For this review, use the dimensioned drawing (mm, ordinates from the lowest corner) and the shaded views. A direction names the side the tool comes from. Give positions to 0.01 mm unless a question says otherwise; leave off trailing zeros. Order: outer loops, then holes, each group sorted by start corner. A loop starts at its lowest first (then second) coordinate and runs counter-clockwise, first axis right, second up.
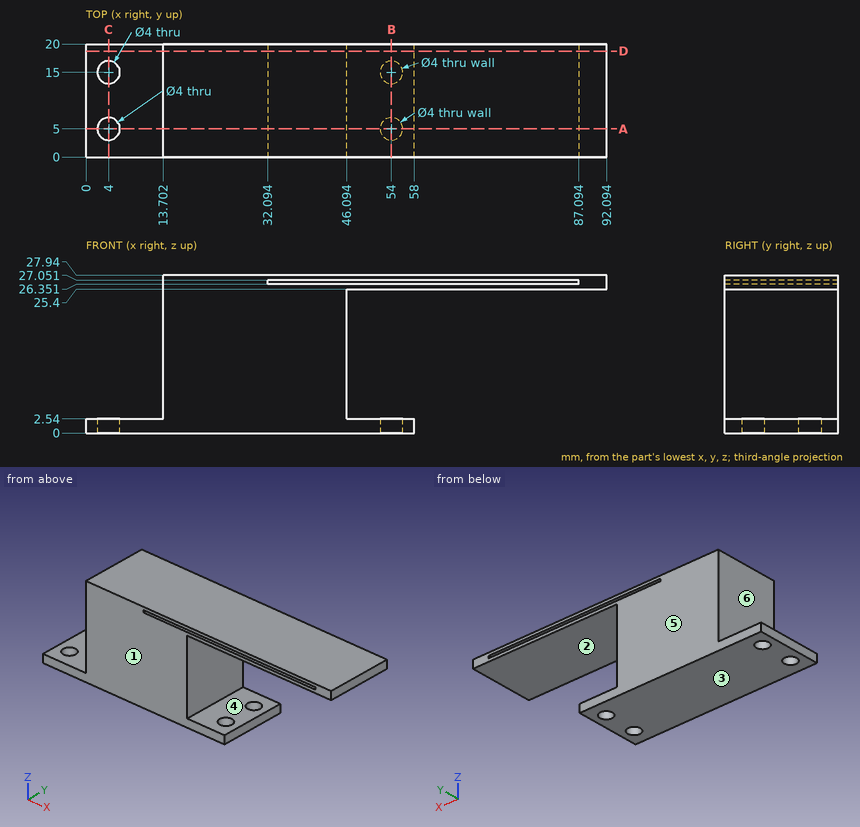
1. For line 1 along Y through (x, z) = (54, 0.5); line 2 along Z through (x, y) = (53.5, 7); line 3 along Z through (x, y) = (62, 13.25), list the stretches that pass through material, from the lowest coordinate up.
Recorded:
line 1: y = 0 to 3, 7 to 13, 17 to 20
line 2: z = 0 to 2.54, 25.4 to 26.35, 27.05 to 27.94
line 3: z = 25.4 to 26.35, 27.05 to 27.94
2. For pin 1 (1.3 mm diameter, centred on y = 6.5, z = 1, fed in from +X); pin 2 (6 mm diameter, centred on x = 78.5, y = 7.5, fed in from -Z); pin 3 (1.5 mm diameter, centred on y = 14, z = 15, fed in from +X); pin 4 (10 mm diameter, centred on x = 52.5, y = 8, fed in from -Z), all flat-tipped, find the tip position at first contact; note any pin that passes through.
Recorded:
pin 1: stops at x = 58
pin 2: stops at z = 25.4
pin 3: stops at x = 46.09
pin 4: stops at z = 0
3. Take a section at B-B (x = 54). State the section outline as (y, z) points, then the cut area to 3 significant figures.
Recorded:
outline: (0, 0) - (3, 0) - (3, 2.54) - (0, 2.54) - close; (0, 25.4) - (20, 25.4) - (20, 26.35) - (0, 26.35) - close; (0, 27.05) - (20, 27.05) - (20, 27.94) - (0, 27.94) - close; (7, 0) - (13, 0) - (13, 2.54) - (7, 2.54) - close; (17, 0) - (20, 0) - (20, 2.54) - (17, 2.54) - close
area: 67.3 mm2
4. Draft analysis for pull direction Z (two halves, no side actions). For the marked faces 1, 2 and 3, state which applies: pulls with the +Z half, pulls with the -Z half, needs draft (parallel to the pull), parting line crosses it, or undercut.
Recorded:
face 1: needs draft
face 2: undercut
face 3: pulls with the -Z half
5. Machinability: for the marked faces 4, 5 and 6, which of the approach directions +Z, -Z, +X, -X, +Y, -Y give a long, thin tool a straight path to every point of the face, cutting with its end or side? Answer none if there is none.
Recorded:
face 4: +X, +Y, -Y
face 5: +Z, -Z, +X, -X, +Y
face 6: +Z, -X, +Y, -Y
6. Take a section at C-C (x = 4). State the section outline as (y, z) points.
Recorded:
outline: (0, 0) - (3, 0) - (3, 2.54) - (0, 2.54) - close; (7, 0) - (13, 0) - (13, 2.54) - (7, 2.54) - close; (17, 0) - (20, 0) - (20, 2.54) - (17, 2.54) - close
7. Take a section at A-A (y = 5). State the section outline as (x, z) points, then the cut area to 3 significant figures.
Recorded:
outline: (0, 0) - (2, 0) - (2, 2.54) - (0, 2.54) - close; (6, 0) - (52, 0) - (52, 2.54) - (46.09, 2.54) - (46.09, 25.4) - (92.09, 25.4) - (92.09, 27.94) - (13.7, 27.94) - (13.7, 2.54) - (6, 2.54) - close; (56, 0) - (58, 0) - (58, 2.54) - (56, 2.54) - close; hole (32.09, 26.35) - (87.09, 26.35) - (87.09, 27.05) - (32.09, 27.05) - close
area: 1,030 mm2
8. Take a section at D-D (y = 18.75). State the section outline as (x, z) points, then the cut area to 3 significant figures.
Recorded:
outline: (0, 0) - (58, 0) - (58, 2.54) - (46.09, 2.54) - (46.09, 25.4) - (92.09, 25.4) - (92.09, 27.94) - (13.7, 27.94) - (13.7, 2.54) - (0, 2.54) - close; hole (32.09, 26.35) - (87.09, 26.35) - (87.09, 27.05) - (32.09, 27.05) - close
area: 1,050 mm2
